Read the model definition and answer for the solid it produces. Units are mm, in the model's axes. A direction names the side the tool comes from. Give positions to 0.01 mm unless a question says otherwise; leave off trailing zeros. Order: outer loops, then holes, each group sorted by start corner. A loop starts at its lowest first (then second) coordinate and runs counter-clockwise, first axis right, second up. Notation, with made-up numbers: M 5,40.5 L 36,40.5 A17 cw 36,73.5 Z; hole C -19,30 d9. An arc over 180 degrees is marked long. One line per item, written item: value.
Autodesk Inventor part; units mm, degrees
ref_plane "YZ Plane" through (0, 0, 0) normal (1, 0, 0) x (0, 1, 0)
ref_plane "XZ Plane" through (0, 0, 0) normal (0, 1, 0) x (-1, 0, 0)
ref_plane "XY Plane" through (0, 0, 0) normal (0, 0, 1) x (1, 0, 0)
sketch "Эскиз1" plane through (0, 0, 0) normal (0, 0, 1) x (1, 0, 0)
  arc A0 (-25, 43.3013) -> (25, 43.3013) centre (0, 0) ccw
  circle A1 centre (0, 0) radius 12
  line L0 (-50, 0) -> (50, 0) construction
  line L1 (0, 0) -> (-24.9984, -43.3022) construction
  line L2 (0, 0) -> (25.0049, -43.3022) construction
  circle A2 centre (0, 0) radius 33 construction
  circle A3 centre (-16.499, -28.5794) radius 9
  circle A4 centre (16.4989, -28.5795) radius 9
  arc A5 (-28.5669, -16.606) -> (-28.0784, -10.5643) centre (-33.4841, -13.1678) ccw
  arc A6 (-26.1975, -14.6174) -> (-26.1978, -14.6176) centre (-16.499, -28.5794) ccw
  arc A7 (-28.5357, -16.5745) -> (-24.9984, -43.3022) centre (-16.499, -28.5794) ccw
  line L3 (0, 0) -> (0, 75)
  arc A8 (20, 75) -> (-20, 75) centre (0, 75) ccw
  arc A9 (10, 75) -> (-10, 75) centre (0, 75) ccw
  line L4 (0, 75) -> (0, 41)
  arc A10 (-20, 41) -> (20, 41) centre (0, 41) ccw construction
  arc A11 (-10, 41) -> (10, 41) centre (0, 41) ccw
  line L5 (-10, 75) -> (-10, 41)
  line L6 (10, 75) -> (10, 41)
  line L7 (0, 21) -> (-26, 21) construction
  line L8 (0, 21) -> (26, 21) construction
  line L9 (-28.0784, -10.5643) -> (28.0784, -10.5643) construction
  arc A12 (28.0091, -10.7467) -> (29.5474, -17.6828) centre (33.4989, -13.1678) ccw
  arc A13 (-0.4419, -29.9967) -> (0.0837, -32.9999) centre (16.4989, -28.5795) ccw
  arc A14 (24.9984, -43.3022) -> (28.5357, -16.5746) centre (16.4989, -28.5795) ccw
  arc A15 (-25, 43.3013) -> (-20, 51.9615) centre (-30, 51.9615) ccw
  arc A16 (20, 51.9615) -> (25, 43.3013) centre (30, 51.9615) ccw
  arc A17 (20, 24.8998) -> (21.6667, 20.7498) centre (26, 24.8998) ccw
  arc A18 (-21.6667, 20.7498) -> (-20, 24.8998) centre (-26, 24.8998) ccw
  arc A19 (-21.4243, 21) -> (-27.753, -11.3916) centre (0, 0) ccw
  arc A20 (27.8299, -11.2025) -> (21.4243, 21) centre (0, 0) ccw
  arc A21 (-24.9984, -43.3022) -> (24.9984, -43.3022) centre (0, 0) ccw
  line L10 (-20, 75) -> (-20, 51.9615)
  line L11 (20, 75) -> (20, 51.9615)
  line L12 (20, 51.9615) -> (20, 24.8998)
  line L13 (-20, 51.9615) -> (-20, 24.8998)
  dimension "d0" = 100
  dimension "d1" = 24
  dimension "d2" = 66
  dimension "d3" = 18
  dimension "d4" = 18
  dimension "d7" = 12
  dimension "d10" = 75
  dimension "d11" = 20
  dimension "d12" = 10
  dimension "d13" = 34
  dimension "d14" = 20
  dimension "d15" = 10
  dimension "d24" = 26
  dimension "d25" = 26
  dimension "d29" = 12
  dimension "d30" = 20
  dimension "d31" = 20
  dimension "d32" = 17
  dimension "d37" = 21
  dimension "d38" = 31.5643
  dimension "d40" = 34.1678
  dimension "d66" = 12
  dimension "d67" = 12
  dimension "d68" = 30
  dimension "d69" = 30
  dimension "d70" = 30.004
  dimension "d71" = 150.002
  dimension "d72" = 13.4989
  dimension "d73" = 9.5474
  dimension "d74" = 8.0784
  dimension "d75" = 8.0091
  dimension "d76" = 5.0049
  dimension "d77" = 0
  dimension "d78" = 20.4419
  dimension "d79" = 46.1975
  dimension "d80" = 46.1978
  dimension "d81" = 47.753
  dimension "d82" = 48.0784
extrude "Выдавливание1" add sketch "Эскиз1" along normal blind 10 contours A15 L13 A18 A19 A5 A6 A0 | A14 A12 A20 A17 L12 A16 A0 | A12 A14
extrude "Выдавливание2" add sketch "Эскиз1" along normal blind 15 contours A6 A5 A19 A18 L13 L10 A8 L11 L12 A17 A20 A12 A14 A0 | A6 | A19 A5 | A12 A20
properties part number "лаб,2_2"
1) Find section A-A, the plane y = 0. Write down the section's boundary in (x, z).
Reported:
outline: M -50,0 L -12,0 L -12,15 L -30,15 L -30,10 L -50,10 Z; M 12,0 L 50,0 L 50,10 L 30,10 L 30,15 L 12,15 Z
2) Which of the six approach directions +Z, -Z, +X, -X, +Y, -Y give full straight-line access (tool end or side, diameter ignored) to faces 4 (the face through (0, 24, 15)), 5 (the face through (27.71, -14.75, 12.46)), 6 (the face through (0, 85, 7)), 7 (the face through (-33.32, -31.05, 12.46)), 8 (the face through (20, 56, 9))?
Reported:
face 4: +Z, +X, -X, +Y, -Y
face 5: +Z, +X
face 6: +Z, -Z
face 7: +Z, -X
face 8: +Z, +X, +Y
3) Find section B-B, the plane x = 0. Write down the section's boundary in (y, z), plus the area to 4 significant figures.
Reported:
outline: M -50,0 L -12,0 L -12,15 L -50,15 Z; M 12,0 L 31,0 L 31,15 L 12,15 Z; M 85,0 L 95,0 L 95,15 L 85,15 Z
area: 1,005 mm^2
4) Find section D-D, the plane x = -38. Write down the section's boundary in (y, z), plus the area to 3 significant figures.
Reported:
outline: M -32.5,0 L 32.5,0 L 32.5,10 L -32.5,10 Z
area: 650 mm^2
5) Consider probe 1 along Y at (x, z) = (-0.5, 4); probe 2 along X at (y, z) = (57.5, 3); probe 3 along X at (y, z) = (0, 6). Determine where each line is inside the solid, lowest interval first.
Reported:
probe 1: y = -50 to -11.99, 11.99 to 31.01, 84.99 to 94.99
probe 2: x = -20 to -10, 10 to 20
probe 3: x = -50 to -12, 12 to 50
6) Each of these flat-tipped pins is pushed along its axis until it touches: pin 1 Ø24 at (x, y) = (-34, 15) entering from +Z; pin 2 Ø7.5 at (y, z) = (50.5, 9.5) entering from +X; pin 3 Ø6 at (y, z) = (11, 4.5) entering from +X; pin 4 Ø9 at (x, y) = (38.5, -3.5) entering from +Z. Where does it stop, or does it pass through?
Reported:
pin 1: stops at z = 15
pin 2: stops at x = 21.47
pin 3: stops at x = 49.36
pin 4: stops at z = 10
7) Determine the mould class of faces 1 (the face through (20.444, 22.634, 12.465)), 2 (the face through (-29.52, 5.34, 12.46)), 3 (the face through (-1, 24, 0)) for opening direction Y: +Y half, -Y half, draft (parallel to the pull), parting line (faces both ways), or undercut.
Reported:
face 1: +Y half
face 2: undercut
face 3: draft
8) Find section C-C, the plane z = 2.5. Write down the section's boundary in (x, y), plus the area to 3 significant figures.
Reported:
outline: M -25,43.3 A50 ccw long 25,43.3 A10 cw 20,51.96 L 20,75 A20 ccw -20,75 L -20,51.96 A10 cw Z; hole C -16.5,-28.58 d18; hole C 0,0 d24; hole M -10,41 A10 ccw 10,41 L 10,75 A10 ccw -10,75 Z; hole C 16.5,-28.58 d18
area: 7,590 mm^2
